from build123d import *

# Parameters (mm, degrees)
CROQUIS1_R              = 1.5
CROQUIS1_R_2            = 10
SALIENTE_EXTRUIR1_DEPTH = 5


with BuildPart() as part:
    # Croquis1 → Saliente-Extruir1 (new body)
    with BuildSketch(Plane.XY):
        Polygon((0, 0), (9.25, 0), (9.25, 9), (5.75, 9), (5.75, 12), (9.25, 12), (9.25, 15), (12.25, 15), (12.25, 12), (15.75, 12), (15.75, 9), (12.25, 9), (12.25, 0), (17.5, 0), (17.5, -5), (32.5, -5), (32.5, 0), (37.75, 0), (37.75, 9), (34.25, 9), (34.25, 12), (37.75, 12), (37.75, 15), (40.75, 15), (40.75, 12), (44.25, 12), (44.25, 9), (40.75, 9), (40.75, 0), (50, 0), (50, 72.5), (40, 72.5), (40, 77.5), (10, 77.5), (10, 72.5), (0, 72.5), align=None)
        with Locations((25, 75)):
            Circle(CROQUIS1_R, mode=Mode.SUBTRACT)
        with Locations((25, 47.5)):
            Circle(CROQUIS1_R_2, mode=Mode.SUBTRACT)
        with Locations((25, 62.5)):
            Circle(CROQUIS1_R, mode=Mode.SUBTRACT)
        with Locations((37.990381057, 40)):
            Circle(CROQUIS1_R, mode=Mode.SUBTRACT)
        with Locations((12.009618943, 40)):
            Circle(CROQUIS1_R, mode=Mode.SUBTRACT)
    extrude(amount=SALIENTE_EXTRUIR1_DEPTH)


solid = part.part
The listing builds one solid part. Answer for the finished solid, in the listing's coordinates (mm). A direction names the side the tool comes from. Round coordinates to 2 decimals unless told otherwise and drop trailing zeros. Loops run counter-clockwise (first coordinate to the right, second up) from the corner with the lowest first, then second, coordinate; pieces in that order, holes last. Notation, with made-up numbers: M -12.5,1 L 11.5,1 A6 ccw 11.5,7 Z; hole C 68,-39 d10. An arc over 180 degrees is marked long. Write each question's results on one line, items separated by ' | '. Start each with the question number.
1) Straight lines are drawn through the part: probe 1 along Y at (x, z) = (25, 1); probe 2 along X at (y, z) = (75, 1.9); probe 3 along Y at (x, z) = (20.5, 4.6). For each, find the intervals that lie inside material, in ascending order.
2) Find section C-C on x = 25. Write down the section's boundary in (y, z).
3) Which of the six approach directions +Z, -Z, +X, -X, +Y, -Y give full straight-line access (tool end or side, diameter ignored) to faces 4 (the flat face through (34.25, 10, 2)), 5 (the flat face through (12.25, 14, 2)), 6 (the flat face through (17.5, -2, 2)), 7 (the flat face through (32.5, -3, 2))?
4) Find section A-A on y = 75. Write down the section's boundary in (x, z), plus the area to 3 significant figures.
5) Each of these flat-tipped pins is pushed along its axis until it touches: pin 1 (1 mm diameter, centred on x = 35.5, z = 3, fed in from -Y); pin 2 (2.5 mm diameter, centred on x = 25, y = 75, fed in from +Z). Where does it stop, or does it pass through?
6) Find section D-D on x = 19.5. Write down the section's boundary in (y, z), plus the area to 3 significant figures.
7) Determine the mould class of faces 1 (the flat face through (15, 0, 2)), 2 (the flat face through (9.25, 4, 2)), 3 (the flat face through (5.75, 10, 2)) for opening direction Y: pulls with the +Y half, pulls with the -Y half, needs draft (parallel to the pull), parting line crosses it, or undercut.
8) Find section B-B on y = 13.5. Write down the section's boundary in (x, z), plus the area to 3 significant figures.
Final values:
1) probe 1: -5 to 37.5, 57.5 to 61, 64 to 73.5, 76.5 to 77.5 | probe 2: 10 to 23.5, 26.5 to 40 | probe 3: -5 to 38.57, 56.43 to 77.5
2) outline: M -5,0 L 37.5,0 L 37.5,5 L -5,5 Z; M 57.5,0 L 61,0 L 61,5 L 57.5,5 Z; M 64,0 L 73.5,0 L 73.5,5 L 64,5 Z; M 76.5,0 L 77.5,0 L 77.5,5 L 76.5,5 Z
3) face 4: +Z, -Z | face 5: +Z, -Z, -Y | face 6: +Z, -Z, -X, -Y | face 7: +Z, -Z, +X, -Y
4) outline: M 10,0 L 23.5,0 L 23.5,5 L 10,5 Z; M 26.5,0 L 40,0 L 40,5 L 26.5,5 Z | area: 135 mm²
5) pin 1: y = 0 | pin 2: through
6) outline: M -5,0 L 39.15,0 L 39.15,5 L -5,5 Z; M 55.85,0 L 77.5,0 L 77.5,5 L 55.85,5 Z | area: 329 mm²
7) face 1: pulls with the -Y half | face 2: needs draft | face 3: undercut
8) outline: M 0,0 L 9.25,0 L 9.25,5 L 0,5 Z; M 12.25,0 L 37.75,0 L 37.75,5 L 12.25,5 Z; M 40.75,0 L 50,0 L 50,5 L 40.75,5 Z | area: 220 mm²
